```python
from build123d import *

# Parameters (mm, degrees)
SKETCH2_W           = 30
SKETCH2_H           = 30
BOSS_EXTRUDE1_DEPTH = 2


with BuildPart() as part:
    # Sketch2 → Boss-Extrude1 (new body)
    with BuildSketch(Plane(origin=(0, 0, 0), x_dir=(1, 0, 0), z_dir=(0, 1, 0))):
        Rectangle(SKETCH2_W, SKETCH2_H)
    extrude(amount=BOSS_EXTRUDE1_DEPTH)

    # Sweep1: sweep along a path in Sketch13
    with BuildLine(Plane.XY) as sweep1_path:
        Line((15, 2), (5, 12))
    # Sketch12 → Sweep1 (sweep)
    with BuildSketch(Plane(origin=(0, 2, 0), x_dir=(1, 0, 0), z_dir=(0, 1, 0))):
        with BuildLine():
            Line((-0.864419204, 11.616439262), (-1.728595106, 12.119629097))
            ThreePointArc((-1.728595106, 12.119629097), (-5, 0), (-1.728595106, -12.119629097))
            Line((-1.728595106, -12.119629097), (-0.864419204, -11.616439262))
            ThreePointArc((-0.864419204, -11.616439262), (-4, 0), (-0.864419204, 11.616439262))
        make_face()
        with BuildLine():
            Line((-2.518797551, 12.579745882), (-3.382973453, 13.082935717))
            ThreePointArc((-3.382973453, 13.082935717), (-6.9144, 0), (-3.382973453, -13.082935717))
            Line((-3.382973453, -13.082935717), (-2.518797551, -12.579745882))
            ThreePointArc((-2.518797551, -12.579745882), (-5.9144, 0), (-2.518797551, 12.579745882))
        make_face()
    sweep(path=sweep1_path.line)


solid = part.part
```
Design review of the part built by this model. Coordinates are the model's own, in mm. Round coordinates to 2 decimals unless told otherwise and drop trailing zeros. Write each loop counter-clockwise with the first axis right and the second up, starting at its lowest first coordinate (ties: lowest second). Pieces come first, ordered by that corner, then holes.
Item 1: For probe 1 along Y at (x, z) = (-9, -5.75); probe 2 along Y at (x, z) = (-10, 1.75); probe 3 along Y at (x, z) = (2.5, -8.5), list the stretches that pass through material, from the lowest coordinate up.
Item 2: We need section A-A on y = 1.5. Write out the cut boundary in (x, z), and give its area (3 significant figures).
Item 3: We need section B-B on x = -0.5. Write out the cut boundary in (y, z).
Item 4: We need section C-C on x = -9. State how many separate pieces and enclosed holes the cut face has, and give its area (3 significant figures).
Item 5: Clearance check with flat-ended pins moving along their axes: pin 1 Ø1 at (y, z) = (10.5, -2.5) entering from +X; pin 2 Ø3 at (y, z) = (6.5, 11.5) entering from -X; pin 3 Ø0.6 at (y, z) = (1, 3.5) entering from -X. State where each tip first meets the part, or that it passes through.
Item 6: The part is to be moulded in two halves that separate along Y. For faces 1 (the flat face through (0, 2, 0)), 2 (the flat face through (-15, 1, 0)), 3 (the flat face through (-7.9, 7, -12.8)), say which applies: +Y half, -Y half, draft (parallel to the pull), parting line (faces both ways), or undercut.
Returned:
1. probe 1: y = 0 to 2, 4.73 to 5.76, 6.7 to 7.73
1. probe 2: y = 0 to 2, 5.14 to 6.15, 7.06 to 8.07
1. probe 3: y = 0 to 2
2. outline: (-15, -15) - (15, -15) - (15, 15) - (-15, 15) - close
2. area: 900 mm2
3. outline: (0, -15) - (2, -15) - (2, 15) - (0, 15) - close
4. separate pieces: 3
4. enclosed holes: 0
4. area: 112 mm2
5. pin 1: stops at x = -11.86
5. pin 2: stops at x = -10.39
5. pin 3: stops at x = -15
6. face 1: undercut
6. face 2: draft
6. face 3: +Y half
